```python
from build123d import *

# Parameters (mm, degrees)
F0_R     = 2
F1_DEPTH = 25
F3_DEPTH = 1
F4_R     = 3.55
F5_DEPTH = 7


with BuildPart() as f1:
    # F0 (on Front) → F1 (new body)
    with BuildSketch(Plane.XZ):
        with BuildLine():
            Line((27.5634530751, 33.6863230431), (27.700783795, -35.983503393))
            ThreePointArc((27.700783795, -35.983503393), (-1.0310012543, -61.2900569115), (-27.5634530751, -33.6863230431))
            Line((-27.5634530751, -33.6863230431), (-27.700783795, 35.983503393))
            ThreePointArc((-27.700783795, 35.983503393), (-24.1975782347, 44.5411756868), (-32.7105452322, 40.9306913446))
            Line((-32.7105452322, 40.9306913446), (-32.5587658259, -36.0691590645))
            Line((-32.5587658259, -36.0691590645), (-32.5587658259, -66.3139410643))
            ThreePointArc((-32.5587658259, -66.3139410643), (-31.0942997319, -69.8494749702), (-27.5587658259, -71.3139410643))
            Line((-27.5587658259, -71.3139410643), (27.700708785, -71.3139410643))
            ThreePointArc((27.700708785, -71.3139410643), (31.236242691, -69.8494749702), (32.700708785, -66.3139410643))
            Line((32.700708785, -66.3139410643), (32.700708785, -35.9405218755))
            Line((32.700708785, -35.9405218755), (32.5535875558, 38.696169135))
            ThreePointArc((32.5535875558, 38.696169135), (24.0111011252, 42.2148712597), (27.5634530751, 33.6863230431))
        make_face()
        with Locations((-24.4080040093, -63.1631792477)):
            Circle(F0_R, mode=Mode.SUBTRACT)
        with Locations((24.4080040093, -63.1631792477)):
            Circle(F0_R, mode=Mode.SUBTRACT)
    extrude(amount=F1_DEPTH)

    # F2 (on face) → F3 (join)
    with BuildSketch(Plane.XZ.offset(25)):
        with BuildLine():
            Line((-26.6844767994, 27.7107327074), (-27.6844767994, 27.7107327074))
            Line((-27.6844767994, 27.7107327074), (-27.6844767994, -2.2892672926))
            Line((-27.6844767994, -2.2892672926), (-26.6844767994, -2.2892672926))
            ThreePointArc((-26.6844767994, -2.2892672926), (-24.5631564558, -1.4105876361), (-23.6844767994, 0.7107327074))
            Line((-23.6844767994, 0.7107327074), (-23.6844767994, 24.7107327074))
            ThreePointArc((-23.6844767994, 24.7107327074), (-24.5631564558, 26.832053051), (-26.6844767994, 27.7107327074))
        make_face()
        with BuildLine():
            Line((26.6844767994, -2.2892672926), (27.6844767994, -2.2892672926))
            Line((27.6844767994, -2.2892672926), (27.6844767994, 27.7107327074))
            Line((27.6844767994, 27.7107327074), (26.6844767994, 27.7107327074))
            ThreePointArc((26.6844767994, 27.7107327074), (24.5631564558, 26.832053051), (23.6844767994, 24.7107327074))
            Line((23.6844767994, 24.7107327074), (23.6844767994, 0.7107327074))
            ThreePointArc((23.6844767994, 0.7107327074), (24.5631564558, -1.4105876361), (26.6844767994, -2.2892672926))
        make_face()
        with BuildLine():
            Line((0.1186772118, -55.3139410643), (-17.0913840546, -55.3139410643))
            ThreePointArc((-17.0913840546, -55.3139410643), (-8.994310893, -59.7709375988), (0.1186772118, -61.3139410643))
            Line((0.1186772118, -61.3139410643), (0.1186772118, -55.3139410643))
        make_face()
        with BuildLine():
            Line((17.3287384782, -55.3139410643), (0.1186772118, -55.3139410643))
            Line((0.1186772118, -55.3139410643), (0.1186772118, -61.3139410643))
            ThreePointArc((0.1186772118, -61.3139410643), (9.2316653166, -59.7709375988), (17.3287384782, -55.3139410643))
        make_face()
    extrude(amount=-F3_DEPTH)

    # F4 (on face) → F5 (cut)
    with BuildSketch(Plane.XZ.offset(25)):
        with Locations((-24.4080040093, -63.1631792477)):
            Circle(F4_R)
        with Locations((24.4080040093, -63.1631792477)):
            Circle(F4_R)
    extrude(amount=-F5_DEPTH, mode=Mode.SUBTRACT)


solid = f1.part
```
Can you work these out from the model? Positions are in its coordinate system, mm. A direction names the side the tool comes from. Round coordinates to 2 decimals unless told otherwise and drop trailing zeros. Loops run counter-clockwise (first coordinate to the right, second up) from the corner with the lowest first, then second, coordinate; pieces in that order, holes last. Notation, with made-up numbers: M 32.5,20 L 78.5,20 A29 cw 78.5,47 Z; hole C -27.5,-36.75 d5. An arc over 180 degrees is marked long. Write item = value, one per line. Start each with the question number.
(1) Suppose I cut it at A-A on x = 25. Write out the boundary of the cut face in (y, z).
(2) I need wall thicknesses on line 1 along Z through (x, y) = (-25, -17.25); line 2 along Z through (x, y) = (25.5, -23); line 3 along X through (y, z) = (-14, -27.5). Which ranges of each line are inside material? Lowest first, please.
(3) Suppose I cut it at C-C on y = -19.5. Write out the boundary of the cut face in (x, z), plus the area to 3 significant figures.
(4) Suppose I cut it at D-D on z = 5. Write out the boundary of the cut face in (x, y).
(5) If we mould it in two halves opening along Z, with no side actions, what happens to faces 5 (the face through (-22, 0, -51)), 6 (the face through (-31.133, -12.325, -69.81)), 7 (the face through (-0.44, -12.32, -61.31))? For each: released by +Z, released by -Z, zero draft, split by the parting line, or undercut.
(6) I'm going to push flat-ended pins straight in: P1, Ø2, axis at x = -23, z = -63.5, coming from the -Y side; P2, Ø12.5, axis at y = -12, z = -49.5, coming from the -X side; P3, Ø2, axis at x = 25, z = 19, coming from the +Y side. Where does each tip first touch, or does it pass through?
(7) Suppose I cut it at B-B on z = -37.5. Write out the boundary of the cut face in (x, y).
(8) Which directions (+Z, -Z, +X, -X, +Y, -Y) give clear straight access to the entire face, cutting with the end or side of a thin tool? Please do faces 1 (the face through (26, -18, -65)), 2 (the face through (26, -24, 13)), 3 (the face through (-32.559, -12, -51)), 4 (the face through (-24.54, -24.51, 26.81)).
Answer block:
q1.outline = M -25,-71.31 L 0,-71.31 L 0,-65.07 L -18,-65.07 L -18,-66.66 L -25,-66.66 Z; M -25,-59.66 L -18,-59.66 L -18,-61.25 L 0,-61.25 L 0,-45.77 L -25,-45.77 Z; M -25,-1.77 L -24,-1.77 L -24,27.19 L -25,27.19 Z; M -25,34.39 L 0,34.39 L 0,42.99 L -25,42.99 Z
q2.line_1 = -71.31 to -65.07, -61.25 to -45.27, 36.78 to 45.18
q2.line_2 = -71.31 to -66.54, -59.79 to -44.68, 34.13 to 43.25
q2.line_3 = -32.58 to -27.58, 27.68 to 32.68
q3.outline = M -32.71,40.93 L -32.56,-36.07 L -32.56,-66.31 A5 ccw -27.56,-71.31 L 27.7,-71.31 A5 ccw 32.7,-66.31 L 32.7,-35.94 L 32.55,38.7 A5 ccw long 27.56,33.69 L 27.7,-35.98 A27.68 cw -27.56,-33.69 L -27.7,35.98 A5 ccw long Z; hole C -24.41,-63.16 d7.1; hole C 24.41,-63.16 d7.1
q3.area = 2,020 mm²
q4.outline = M -32.64,-25 L -23.68,-25 L -23.68,-24 L -27.64,-24 L -27.64,0 L -32.64,0 Z; M 23.68,-25 L 32.62,-25 L 32.62,0 L 27.62,0 L 27.62,-24 L 23.68,-24 Z
q5.face_5 = zero draft
q5.face_6 = released by -Z
q5.face_7 = undercut
q6.P1 = -18
q6.P2 = -32.56
q6.P3 = -24
q7.outline = M -32.56,-25 L -27.29,-25 L -27.29,0 L -32.56,0 Z; M 27.53,-25 L 32.7,-25 L 32.7,0 L 27.53,0 Z
q8.face_1 = -Y
q8.face_2 = +Y
q8.face_3 = -Z, -X, +Y, -Y
q8.face_4 = +Y, -Y
